from build123d import *

# Parameters (mm, degrees)
F0_R     = 18.5
F1_DEPTH = 2
F2_R     = 12.5
F3_DEPTH = 5
F4_R     = 10.5
F5_DEPTH = 25
F6_R     = 1
F7_R     = 0.99999
F8_R     = 0.99999


# Not quite as in the source:
# - a fillet or chamfer is up to 0.001 mm smaller than in the source, because OpenCascade refuses the exact size


with BuildPart() as f1:
    # F0 (on Top) → F1 (new body)
    with BuildSketch(Plane.XY):
        Circle(F0_R)
    extrude(amount=F1_DEPTH)

    # F2 (on face) → F3 (join)
    with BuildSketch(Plane.XY.offset(2)):
        Circle(F2_R)
    extrude(amount=F3_DEPTH)

    # F4 (on face) → F5 (cut)
    with BuildSketch(Plane.XY.offset(7)):
        Circle(F4_R)
    extrude(amount=-F5_DEPTH, mode=Mode.SUBTRACT)

    # F6
    f6_edges = [f1.edges().sort_by_distance(p)[0] for p in [
        (-18.5, 0, 0),
        (-10.5, 0, 0),
    ]]
    fillet(f6_edges, radius=F6_R)

    # F7 (radius 1 in the source; OpenCascade refuses exactly that, so slightly less here)
    f7_edges = [f1.edges().sort_by_distance(p)[0] for p in [
        (-12.5, 0, 7),
        (-10.5, 0, 7),
    ]]
    fillet(f7_edges, radius=F7_R)

    # F8 (radius 1 in the source; OpenCascade refuses exactly that, so slightly less here)
    f8_edges = [f1.edges().sort_by_distance(p)[0] for p in [
        (-18.5, 0, 2),
    ]]
    fillet(f8_edges, radius=F8_R)


solid = f1.part
Check sheet for the modelled part. Datum: model origin and axes. Units: mm. A direction names the side the tool comes from. Round coordinates to 2 decimals unless told otherwise and drop trailing zeros. Loops run counter-clockwise (first coordinate to the right, second up) from the corner with the lowest first, then second, coordinate; pieces in that order, holes last. Notation, with made-up numbers: (73.5, 2.5) -> (81.5, 2.5) arc R7 ccw to (81.5, 11.5) -> close; hole circle Ø11 at (40.25, 81). An arc over 180 degrees is marked (long way). Put each result on its own line as item: value. Start each with the question number.
1. Access from +Z, -Z, +X, -X, +Y, -Y to the whole of each face (thin tool, end or side, straight path). Record for faces 1 (the face through (11, -8, 2)), 2 (the face through (4, -11, 0)).
2. Section check C-C (z = 3.5). Enter the section's corners in (x, y).
3. Gauge pin test, flat ends, axial feed: pin 1 (4 mm diameter, centred on x = 13, z = 4.5, fed in from +Y); pin 2 (4 mm diameter, centred on x = 0.5, y = 10, fed in from -Z); pin 3 (1.5 mm diameter, centred on x = 8.5, z = 5.5, fed in from +Y). Record the tip position at first contact, or that the pin passes through.
4. Scan lines: probe 1 along Y at (x, z) = (0, 2.8); probe 2 along Z at (x, y) = (-13.5, 10); probe 3 along Y at (x, z) = (-7, 6). Record each from-to range of solid material in increasing order.
Findings:
1. face 1: +Z
1. face 2: -Z, +X, -X, +Y, -Y
2. outline: circle Ø25 at (0, 0); hole circle Ø21 at (0, 0)
3. pin 1: stops at y = 5.94
3. pin 2: stops at z = 0
3. pin 3: stops at y = 9.81
4. probe 1: y = -12.5 to -10.5, 10.5 to 12.5
4. probe 2: z = 0 to 2
4. probe 3: y = -10.36 to -7.83, 7.83 to 10.36
